Model file for the job. Use its own axes, mm. Face numbers are marked on the shaded views. A direction names the side the tool comes from. Round coordinates to 2 decimals unless told otherwise and drop trailing zeros. Loops run counter-clockwise (first coordinate to the right, second up) from the corner with the lowest first, then second, coordinate; pieces in that order, holes last. Notation, with made-up numbers: (-20, -23.5) -> (3, -23.5) arc R28 ccw to (3, 10.5) -> close; hole circle Ø5 at (14, 19.5). An arc over 180 degrees is marked (long way). Use a Markdown table: item, result.
from build123d import *

# Parameters (mm, degrees)
ESBO_O1_R                = 1.6
RESSALTO_EXTRUS_O1_DEPTH = 3


with BuildPart() as part:
    # Esboço1 → Ressalto-extrusão1 (new body)
    with BuildSketch(Plane.XZ.offset(3)):
        with BuildLine():
            Line((-7.1, -28.6), (7.1, -28.6))
            ThreePointArc((7.1, -28.6), (14.171067812, -25.671067812), (17.1, -18.6))
            Line((17.1, -18.6), (17.1, -6))
            Line((17.1, -6), (7.5, -6))
            Line((7.5, -6), (7.5, 0))
            Line((7.5, 0), (-7.5, 0))
            Line((-7.5, 0), (-7.5, -6))
            Line((-7.5, -6), (-17.1, -6))
            Line((-17.1, -6), (-17.1, -18.6))
            ThreePointArc((-17.1, -18.6), (-14.171067812, -25.671067812), (-7.1, -28.6))
        make_face()
        with Locations(Location((-12.5, -22, 0), (0, 0, 270))):
            Circle(ESBO_O1_R, mode=Mode.SUBTRACT)
        with Locations(Location((12.5, -22, 0), (0, 0, 270))):
            Circle(ESBO_O1_R, mode=Mode.SUBTRACT)
    extrude(amount=-RESSALTO_EXTRUS_O1_DEPTH)


solid = part.part
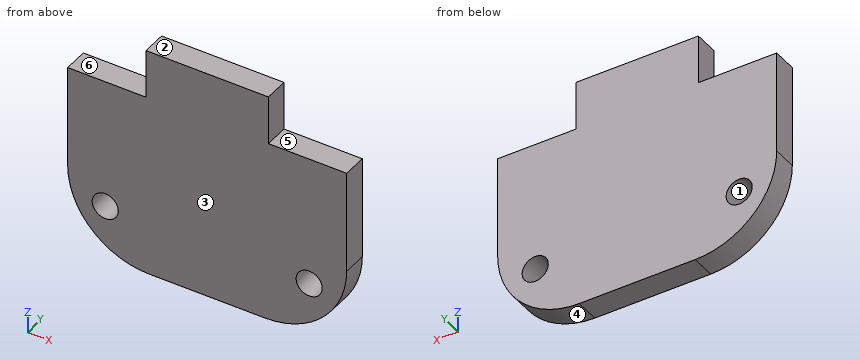
Q1. Band-saw the part on D-D, the plane x = -12. Give the cut face in (y, z), plus the area to 3 significant figures.
Results list:
| item | result |
|---|---|
| outline | (-3, -27.32) -> (0, -27.32) -> (0, -23.52) -> (-3, -23.52) -> close; (-3, -20.48) -> (0, -20.48) -> (0, -6) -> (-3, -6) -> close |
| area | 54.8 mm² |
Q2. Flat gauge pins, fed straight in: pin 1 (1.5 mm diameter, centred on y = -1.5, z = -3, fed in from +X); pin 2 (1 mm diameter, centred on x = 10, y = -1, fed in from -Z); pin 3 (1.5 mm diameter, centred on x = -12, y = -2, fed in from +Z). Where does each tip first touch, or does it go through?
Results list:
| item | result |
|---|---|
| pin 1 | stops at x = 7.5 |
| pin 2 | stops at z = -28.31 |
| pin 3 | stops at z = -6 |
Q3. Pull direction Z, two halves, no side cores. Call the marked faces 1, 2 and 3: released by +Z, released by -Z, zero draft, split by the parting line, or undercut.
Results list:
| item | result |
|---|---|
| face 1 | undercut |
| face 2 | released by +Z |
| face 3 | zero draft |
Q4. Tool access for the marked faces 4, 5 and 6: list every direction of +Z, -Z, +X, -X, +Y, -Y with a clear straight run to the whole face (end or side of a thin tool).
Results list:
| item | result |
|---|---|
| face 4 | -Z, +X, +Y, -Y |
| face 5 | +Z, +X, +Y, -Y |
| face 6 | +Z, -X, +Y, -Y |
Q5. Band-saw the part on A-A, the plane y = -1.25. Give the cut face in (x, z), plus the area to 3 significant figures.
Results list:
| item | result |
|---|---|
| outline | (-17.1, -18.6) arc R10 ccw to (-7.1, -28.6) -> (7.1, -28.6) arc R10 ccw to (17.1, -18.6) -> (17.1, -6) -> (7.5, -6) -> (7.5, 0) -> (-7.5, 0) -> (-7.5, -6) -> (-17.1, -6) -> close; hole circle Ø3.2 at (-12.5, -22); hole circle Ø3.2 at (12.5, -22) |
| area | 804 mm² |
Q6. Band-saw the part on C-C, the plane z = -22. Give the cut face in (x, y).
Results list:
| item | result |
|---|---|
| outline | (-16.5, -3) -> (-14.1, -3) -> (-14.1, 0) -> (-16.5, 0) -> close; (-10.9, -3) -> (10.9, -3) -> (10.9, 0) -> (-10.9, 0) -> close; (14.1, -3) -> (16.5, -3) -> (16.5, 0) -> (14.1, 0) -> close |
Q7. Band-saw the part on B-B, the plane x = 12.5. Give the cut face in (y, z).
Results list:
| item | result |
|---|---|
| outline | (-3, -27.02) -> (0, -27.02) -> (0, -23.6) -> (-3, -23.6) -> close; (-3, -20.4) -> (0, -20.4) -> (0, -6) -> (-3, -6) -> close |
Q8. Drill centre lines: L1, parallel to X at y = -0.65, z = -22; L2, parallel to X at y = -0.35, z = -20.75; L3, parallel to Z at x = -13, y = -1.2. Where is each one in solid material? Low to high. Write a range as from..to.
Results list:
| item | result |
|---|---|
| L1 | x = -16.5..-14.1, -10.9..10.9, 14.1..16.5 |
| L2 | x = -16.87..-13.5, -11.5..11.5, 13.5..16.87 |
| L3 | z = -26.67..-23.52, -20.48..-6 |
